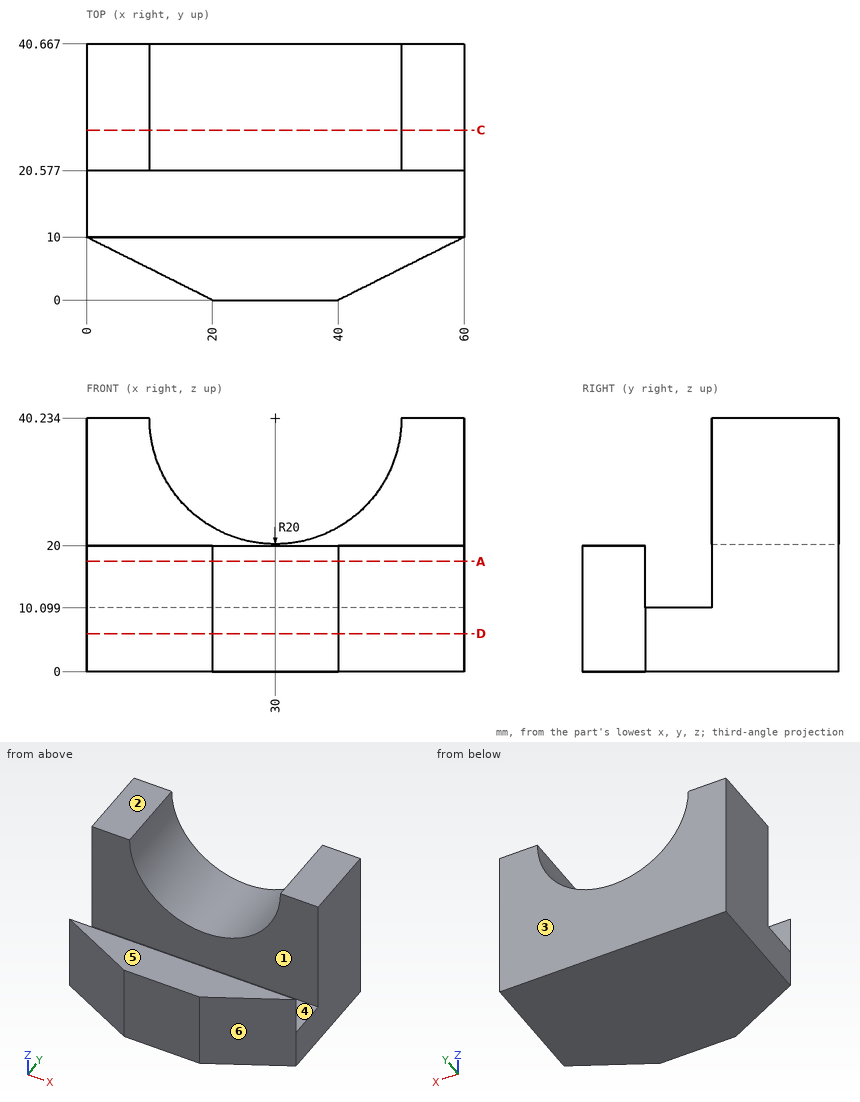
Geometry check sheet. Reference: drawing and pictorial views, mm from the part's lowest x, y, z. A direction names the side the tool comes from. Round coordinates to 2 decimals unless told otherwise and drop trailing zeros. Loops run counter-clockwise (first coordinate to the right, second up) from the corner with the lowest first, then second, coordinate; pieces in that order, holes last. Notation, with made-up numbers: (-39.75, 78.5) - (-21.75, 78.5) arc R26 ccw to (-21.75, 110.5) - close; hole circle Ø1 at (-15.75, 67). An arc over 180 degrees is marked (long way). One line per question, with ' | ' between items. Start each with the question number.
1. Cross-section at C-C on y = 27. Record the cut outline in (x, z) (1 decimal).
2. Depth check by flat-ended pin: pin 1 (10 mm diameter, centred on y = 7.5, z = 20.5, fed in from -X); pin 2 (2 mm diameter, centred on x = 20.5, z = 21.5, fed in from -Y); pin 3 (8 mm diameter, centred on x = 25.5, y = 4, fed in from +Z); pin 4 (1.5 mm diameter, centred on x = 24.5, y = 15, fed in from +Z). Enter the tip coordinate at first touch or a pass-through.
3. Draft check along Y on the marked faces 1, 2, 3 and 4. Enter one of: released by +Y, released by -Y, zero draft, split by the parting line, or undercut.
4. Scan lines: line 1 (Z direction, x = 57, y = 20.5); line 2 (Z direction, x = 33.5, y = 8); line 3 (X direction, y = 5, z = 16). Record each from-to range of solid material in increasing order. Write a range as [from, to].
5. Cross-section at D-D on z = 6. Record the cut outline in (x, y), then the cut area to 3 significant figures.
6. Tool access check on the marked faces 5 and 6. Record the directions out of +Z, -Z, +X, -X, +Y, -Y that give a thin tool (end or side, any length) a straight path to the whole face; none if there is none.
7. Cross-section at A-A on z = 17.5. Record the cut outline in (x, y).
Taken from the geometry:
1) outline: (0, 0) - (60, 0) - (60, 40.2) - (50, 40.2) arc R20 cw to (10, 40.2) - (0, 40.2) - close
2) pin 1: x = 0 | pin 2: y = 20.58 | pin 3: z = 20 | pin 4: z = 10.1
3) face 1: undercut | face 2: zero draft | face 3: released by +Y | face 4: undercut
4) line 1: [0, 10.1] | line 2: [0, 20] | line 3: [10, 50]
5) outline: (0, 10) - (20, 0) - (40, 0) - (60, 10) - (60, 40.67) - (0, 40.67) - close | area: 2,240 mm²
6) face 5: +Z, +X, -X, -Y | face 6: +Z, -Z, +X, -Y
7) outline: (0, 10) - (20, 0) - (40, 0) - (60, 10) - close; (0, 20.58) - (60, 20.58) - (60, 40.67) - (0, 40.67) - close
